from build123d import *

# Parameters (mm, degrees)
SKETCH1_R           = 17.75
BOSS_EXTRUDE1_DEPTH = 12
CUT_EXTRUDE1_DEPTH  = 37


with BuildPart() as part:
    # Sketch1 → Boss-Extrude1 (new body)
    with BuildSketch(Plane(origin=(0, 0, 0), x_dir=(1, 0, 0), z_dir=(0, 1, 0))):
        with BuildLine():
            Line((-85.725, -150.69249853), (24.062600581, -150.69249853))
            Line((24.062600581, -150.69249853), (24.062600581, 0))
            ThreePointArc((24.062600581, 0), (0, 24.062600581), (-24.062600581, 0))
            Line((-24.062600581, 0), (-24.062600581, -21.619479895))
            Line((-24.062600581, -21.619479895), (-85.725, -150.69249853))
        make_face()
        with Locations(Location((0, 0, 0), (0, 0, 270))):
            Circle(SKETCH1_R, mode=Mode.SUBTRACT)
    extrude(amount=BOSS_EXTRUDE1_DEPTH)

    # Sketch3 → Cut-Extrude1 (cut)
    with BuildSketch(Plane.XZ):
        Polygon((14.062600581, 46.322856575), (14.062600581, 29.384281384), (-16.689552863, 29.384281384), (-69.865126015, 140.69249853), (14.062600581, 140.69249853), align=None)
    extrude(amount=-CUT_EXTRUDE1_DEPTH, mode=Mode.SUBTRACT)


solid = part.part
Input: part model. Units: mm. Frame: model coordinates. A direction names the side the tool comes from. Give positions to 0.01 mm unless a question says otherwise; leave off trailing zeros. Loops run counter-clockwise (first coordinate to the right, second up) from the corner with the lowest first, then second, coordinate; pieces in that order, holes last. Notation, with made-up numbers: (78, 79) - (102, 79) arc R20 cw to (102, 93) - close; hole circle Ø4 at (-36, 19). An arc over 180 degrees is marked (long way). Use CSV: the item, a comma, the result in double quotes. Start each with the question number.
Item 1: Contact query for flat-ended pins moving along their axis: P1, Ø3.5, axis at x = -9.5, y = 9, coming from the -Z side; P2, Ø4, axis at x = -46, y = 9.5, coming from the -Z side; P3, Ø8, axis at x = -19, z = 24.5, coming from the -Y side; P4, Ø6, axis at y = 5, z = 7.5, coming from the -X side. Output: stop coordinate, or through.
Item 2: Line query: line 1 (Z direction, x = -0.5, y = 3.5); line 2 (X direction, y = 6.25, z = 0); line 3 (Z direction, x = -11, y = 6). Output: solid intervals per line, ascending.
Item 3: Section C-C on z = 84.5. Return loops of the section in (x, y).
Item 4: Section A-A on x = 0. Return loops of the section in (y, z).
Item 5: Reachability of faces 4 (the flat face through (-24.063, 6, 11)), 5 (the flat face through (-42.905, 5.916, 84.259)), 6 (the flat face through (-35, 12, 63)) from +Z, -Z, +X, -X, +Y, -Y: full face, straight path, thin tool, end or side. Return the list, or none.
Item 6: Mould query, pull axis Z, two halves, no side actions, for faces 1 (the flat face through (24.063, 6, 76)), 2 (the cylindrical face through (-15.747, 5.916, 8.191)), 3 (the cylindrical face through (0.529, 5.916, -24.057)). Classes: pulls with the +Z half, pulls with the -Z half, needs draft (parallel to the pull), parting line crosses it, or undercut.
Item 7: Section B-B on y = 2.25. State how many separate pieces and enclosed holes the cut face has, then the cut area to 3 significant figures.
Item 8: Section D-D on x = -21.5. Return loops of the section in (y, z).
Ans:
1,P1,"stops at z = -22.78"
1,P2,"stops at z = 63.35"
1,P3,"stops at y = 0"
1,P4,"stops at x = -24.06"
2,line 1,"z = -24.06 to -17.74, 17.74 to 29.38, 140.69 to 150.69"
2,line 2,"x = -24.06 to -17.75, 17.75 to 24.06"
2,line 3,"z = -21.4 to -13.93, 13.93 to 29.38, 140.69 to 150.69"
3,outline,"(-54.1, 0) - (-43.02, 0) - (-43.02, 12) - (-54.1, 12) - close; (14.06, 0) - (24.06, 0) - (24.06, 12) - (14.06, 12) - close"
4,outline,"(0, -24.06) - (12, -24.06) - (12, -17.75) - (0, -17.75) - close; (0, 17.75) - (12, 17.75) - (12, 29.38) - (0, 29.38) - close; (0, 140.69) - (12, 140.69) - (12, 150.69) - (0, 150.69) - close"
5,face 4,"-Z, -X, +Y, -Y"
5,face 5,"+Y, -Y"
5,face 6,"+Z, -Z, +X, -X, +Y"
6,face 1,"needs draft"
6,face 2,"undercut"
6,face 3,"pulls with the -Z half"
7,separate pieces,"1"
7,enclosed holes,"2"
7,area,"4,770 mm2"
8,outline,"(0, -10.81) - (12, -10.81) - (12, 39.45) - (0, 39.45) - close; (0, 140.69) - (12, 140.69) - (12, 150.69) - (0, 150.69) - close"
